Read the model definition and answer for the solid it produces. Units are mm, in the model's axes. A direction names the side the tool comes from. Coordinates: 2 decimals unless noted, no trailing zeros. Write each loop counter-clockwise with the first axis right and the second up, starting at its lowest first coordinate (ties: lowest second). Pieces come first, ordered by that corner, then holes.
Item 1: A tool of negligible diameter and unlimited length cuts with its end or side. For faces 1 (the face through (29.859, 94.797, 33.566)), 2 (the face through (-1, 1, 0)), from which of +Z, -Z, +X, -X, +Y, -Y can it reach the whole face along a straight path? Write none if from no direction.
Item 2: This flat-tipped pin is pushed along its axis until it touches: P1, Ø15, axis at x = 26, y = -24.5, coming from the +Z side. Where does it stop, or does it pass through?
Item 3: Section C-C (z = 26.5) is taken. State how many separate pieces and enclosed holes the cut face has, then the cut area to 3 significant figures.
Item 4: Section D-D (x = 13) is taken. Give the vertices of the cut face in (y, z), then the cut area to 3 significant figures.
Item 5: Straight lines are drawn through the part: probe 1 along X at (y, z) = (-54, 14); probe 2 along Y at (x, z) = (10, 13); probe 3 along Y at (x, z) = (27.5, 12.5). For each, find the intervals that lie inside material, in ascending order.
Item 6: Section A-A (x = -3) is taken. Give the vertices of the cut face in (y, z), then the cut area to 3 significant figures.
Item 7: Section B-B (y = -70.5) is taken. Give the vertices of the cut face in (x, z).
Item 8: Determine the mould class of faces 3 (the face through (-1, -100, 32)), 4 (the face through (-45, -1, 32)), 5 (the face through (-21, 0, 34)) for opening direction Y: released by +Y, released by -Y, zero draft, split by the parting line, or undercut.
from build123d import *

# Parameters (mm, degrees)
F0_W        = 90
F0_H        = 200
F1_DEPTH    = 65
F2_W        = 62
F2_H        = 92
F2_W_2      = 30
F2_H_2      = 60
F2_H_3      = 5
F3_DEPTH    = 62
F4_R        = 4
F6_W        = 10
F6_H        = 25
F7_DEPTH    = 62
F8_T4_DEPTH = 90.2885128676
F8_T9_DEPTH = 90.2885128676
F9_R        = 2
F10_R       = 5


# Not quite as in the source:
# - a fillet or chamfer that OpenCascade refuses, or shapes differently, is made with other operations: its cross-section is extruded or revolved along the edge and cut away or added


with BuildPart() as f1:
    # F0 (on Top) → F1 (new body)
    with BuildSketch(Plane.XY):
        Rectangle(F0_W, F0_H)
    extrude(amount=F1_DEPTH)

    # F2 (on face) → F3 (cut)
    with BuildSketch(Plane.XY.offset(65)):
        with Locations((0, 50)):
            Rectangle(F2_W, F2_H)
        with Locations((26, -30)):
            Rectangle(F2_W_2, F2_H_2)
        with Locations((20, -80.5)):
            Rectangle(F2_W_2, F2_H_3)
        with Locations((20, -93.5)):
            Rectangle(F2_W_2, F2_H_3)
        with Locations((-20, -93.5)):
            Rectangle(F2_W_2, F2_H_3)
        with Locations((-20, -80.5)):
            Rectangle(F2_W_2, F2_H_3)
        with BuildLine():
            Line((-12, 0), (-30, 0))
            Line((-30, 0), (-30, -10))
            ThreePointArc((-30, -10), (-28.9453156465, -20.2154821845), (-25.8257569496, -30))
            ThreePointArc((-25.8257569496, -30), (-28.9453156465, -39.7845178155), (-30, -50))
            Line((-30, -50), (-30, -60))
            Line((-30, -60), (-12, -60))
            Line((-12, -60), (-12, -50))
            ThreePointArc((-12, -50), (-13.0546843535, -39.7845178155), (-16.1742430504, -30))
            ThreePointArc((-16.1742430504, -30), (-13.0546843535, -20.2154821845), (-12, -10))
            Line((-12, -10), (-12, 0))
        make_face()
    extrude(amount=-F3_DEPTH, mode=Mode.SUBTRACT)

    # F4
    f4_edges = [f1.edges().sort_by_distance(p)[0] for p in [
        (-31, 96, 34),
        (31, 96, 34),
        (-31, 4, 34),
        (31, 4, 34),
    ]]
    fillet(f4_edges, radius=F4_R)

    # F6 (on face) → F7 (cut, through all)
    with BuildSketch(Plane.XY.offset(65)):
        with Locations((36, 50)):
            Rectangle(F6_W, F6_H)
        Polygon((-30, -60), (-33.5, -60), (-33.5, -75), (-8.5, -75), (-8.5, -60), (-12, -60), align=None)
    extrude(amount=-F7_DEPTH, mode=Mode.SUBTRACT)

    # F8: chamfer of 11 on 2 edges, made by hand


with BuildPart() as f8_tool2:
    # F8_s3 → F8_t4 (new body)
    with BuildSketch(Plane.XY.offset(93.2885128676)):
        Polygon((42, 62.5), (31, 73.5), (31, 62.5), align=None)
    extrude(amount=-F8_T4_DEPTH)

    split(bisect_by=Plane.YZ.offset(41), keep=Keep.BOTTOM)


with BuildPart() as f1_1:
    add(f1.part)

    # F8_t1: cut F8_tool2
    add(f8_tool2.part, mode=Mode.SUBTRACT)


with BuildPart() as f8_tool7:
    # F8_s8 → F8_t9 (new body)
    with BuildSketch(Plane.XY.offset(93.2885128676)):
        Polygon((31, 26.5), (42, 37.5), (31, 37.5), align=None)
    extrude(amount=-F8_T9_DEPTH)

    split(bisect_by=Plane.YZ.offset(41), keep=Keep.BOTTOM)


with BuildPart() as f1_2:
    add(f1_1.part)

    # F8_t6: cut F8_tool7
    add(f8_tool7.part, mode=Mode.SUBTRACT)

    # F9
    f9_edges = [f1_2.edges().sort_by_distance(p)[0] for p in [
        (31, 73.5, 34),
        (41, 63.5, 34),
        (41, 36.5, 34),
        (31, 26.5, 34),
        (-30, 0, 34),
        (-12, 0, 34),
        (-16.174243, -30, 34),
        (-25.825757, -30, 34),
        (-30, -60, 34),
        (-12, -60, 34),
        (-8.5, -75, 34),
        (-33.5, -75, 34),
        (-35, -78, 34),
        (-35, -91, 34),
        (5, -91, 34),
        (5, -78, 34),
        (-5, -91, 34),
        (-5, -78, 34),
        (35, -78, 34),
        (35, -91, 34),
        (-5, -83, 34),
        (-5, -96, 34),
        (35, -96, 34),
        (35, -83, 34),
        (5, -96, 34),
        (5, -83, 34),
        (-35, -83, 34),
        (-35, -96, 34),
    ]]
    fillet(f9_edges, radius=F9_R)

    # F10
    f10_edges = [f1_2.edges().sort_by_distance(p)[0] for p in [
        (-33.5, -60, 34),
        (-8.5, -60, 34),
    ]]
    fillet(f10_edges, radius=F10_R)


solid = f1_2.part
Established:
1. face 1: +Z
1. face 2: -Z, +X, -X, +Y, -Y
2. P1: stops at z = 3
3. separate pieces: 1
3. enclosed holes: 7
3. area: 8,210 mm2
4. outline: (-100, 0) - (100, 0) - (100, 65) - (96, 65) - (96, 3) - (4, 3) - (4, 65) - (0, 65) - (0, 3) - (-60, 3) - (-60, 65) - (-78, 65) - (-78, 3) - (-83, 3) - (-83, 65) - (-91, 65) - (-91, 3) - (-96, 3) - (-96, 65) - (-100, 65) - close
4. area: 2,960 mm2
5. probe 1: x = -45 to -30, -12 to 11, 41 to 45
5. probe 2: y = -100 to -96, -91 to -83, -78 to 4, 96 to 100
5. probe 3: y = -100 to -96, -91 to -83, -78 to -60, 0 to 4.03, 95.97 to 100
6. outline: (-100, 0) - (100, 0) - (100, 65) - (96, 65) - (96, 3) - (4, 3) - (4, 65) - (-100, 65) - close
6. area: 7,300 mm2
7. outline: (-45, 0) - (45, 0) - (45, 65) - (-8.5, 65) - (-8.5, 3) - (-33.5, 3) - (-33.5, 65) - (-45, 65) - close
8. face 3: released by -Y
8. face 4: zero draft
8. face 5: undercut
